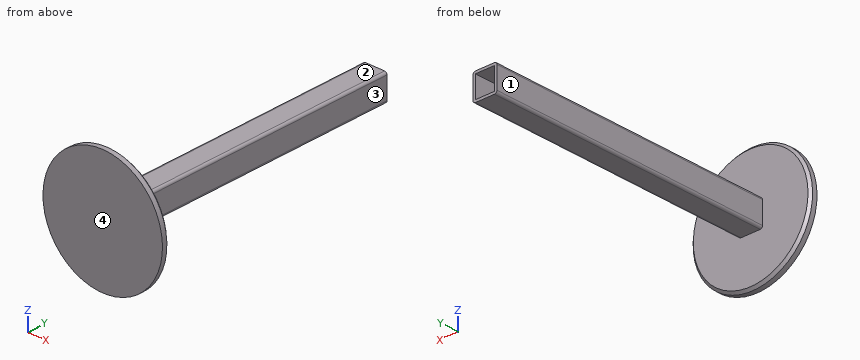
from build123d import *

# Parameters (mm, degrees)
SKETCH1_R           = 250
BOSS_EXTRUDE1_DEPTH = 30
SKETCH2_W           = 100
SKETCH2_H           = 110
BOSS_EXTRUDE2_DEPTH = 1200
CHAMFER1_SIZE       = 10
FILLET1_R           = 10
SKETCH3_W           = 80
SKETCH3_H           = 90
CUT_EXTRUDE1_DEPTH  = 1170


with BuildPart() as part:
    # Sketch1 → Boss-Extrude1 (new body)
    with BuildSketch(Plane(origin=(0, 0, 0), x_dir=(1, 0, 0), z_dir=(0, 1, 0))):
        with Locations(Location((0, 0, 0), (0, 0, 270))):
            Circle(SKETCH1_R)
    extrude(amount=BOSS_EXTRUDE1_DEPTH)

    # Sketch2 → Boss-Extrude2 (add)
    with BuildSketch(Plane(origin=(0, 30, 0), x_dir=(1, 0, 0), z_dir=(0, 1, 0))):
        Rectangle(SKETCH2_W, SKETCH2_H)
    extrude(amount=BOSS_EXTRUDE2_DEPTH)

    # Chamfer1
    chamfer1_edges = [part.edges().sort_by_distance(p)[0] for p in [
        (0, 30, -250),
    ]]
    chamfer(chamfer1_edges, length=CHAMFER1_SIZE)

    # Fillet1
    fillet1_edges = [part.edges().sort_by_distance(p)[0] for p in [
        (-50, 630, -55),
        (-50, 630, 55),
        (50, 630, 55),
        (50, 630, -55),
    ]]
    fillet(fillet1_edges, radius=FILLET1_R)

    # Sketch3 → Cut-Extrude1 (cut)
    with BuildSketch(Plane(origin=(0, 1230, 0), x_dir=(1, 0, 0), z_dir=(0, 1, 0))):
        Rectangle(SKETCH3_W, SKETCH3_H)
    extrude(amount=-CUT_EXTRUDE1_DEPTH, mode=Mode.SUBTRACT)


solid = part.part
CAD build for the part. Positions are in the model's coordinates, mm. Face numbers are marked on the shaded views. A direction names the side the tool comes from. Round coordinates to 2 decimals unless told otherwise and drop trailing zeros. Loops run counter-clockwise (first coordinate to the right, second up) from the corner with the lowest first, then second, coordinate; pieces in that order, holes last.
(1) Cut at B-B (y = 129). Give the cut face in (x, z), plus the area to 3 significant figures.
(2) Cut at C-C (x = 0). Give the cut face in (y, z).
(3) Drop flat-ended pins along their axis: pin 1 (24 mm diameter, centred on x = 6, y = 415.5, fed in from +Z); pin 2 (5 mm diameter, centred on x = -14, z = 106, fed in from +Y). Give the stop position or say it passes through.
(4) Cut at A-A (z = 0). Give the cut face in (x, y).
(5) Which spindle directions (+Z, -Z, +X, -X, +Y, -Y) get a long thin tool onto all of the face, cutting with end or side? Do the marked faces 1, 2, 3 and 4. Say none if no direction does.
(6) Wall check: line 1 along Z through (x, y) = (6, 637.5); line 2 along Y through (x, z) = (106, -78.5); line 3 along X through (y, z) = (317, 46). Give the ranges that are in metal, low to high.
Findings below:
1. outline: (-50, -45) arc R10 ccw to (-40, -55) - (40, -55) arc R10 ccw to (50, -45) - (50, 45) arc R10 ccw to (40, 55) - (-40, 55) arc R10 ccw to (-50, 45) - close; hole (-40, -45) - (40, -45) - (40, 45) - (-40, 45) - close
1. area: 3,710 mm2
2. outline: (0, -250) - (20, -250) - (30, -240) - (30, -55) - (1230, -55) - (1230, -45) - (60, -45) - (60, 45) - (1230, 45) - (1230, 55) - (30, 55) - (30, 240) - (20, 250) - (0, 250) - close
3. pin 1: stops at z = 55
3. pin 2: stops at y = 30
4. outline: (-250, 0) - (250, 0) - (250, 20) - (240, 30) - (50, 30) - (50, 1230) - (40, 1230) - (40, 60) - (-40, 60) - (-40, 1230) - (-50, 1230) - (-50, 30) - (-240, 30) - (-250, 20) - close
5. face 1: +Z, -Z, -X, +Y
5. face 2: +Z, +X, -X, +Y
5. face 3: +Z, -Z, +X, +Y
5. face 4: +Z, -Z, +X, -X, -Y
6. line 1: z = -55 to -45, 45 to 55
6. line 2: y = 0 to 30
6. line 3: x = -49.95 to 49.95
